Source: CAD feature listing. Evaluate the final solid. Frame: model axes, mm. A direction names the side the tool comes from. Round coordinates to 2 decimals unless told otherwise and drop trailing zeros. Loops run counter-clockwise (first coordinate to the right, second up) from the corner with the lowest first, then second, coordinate; pieces in that order, holes last.
(1) Section C-C, the plane y = 86. Return the cut outline in (x, z).
(2) Section A-A, the plane x = 155. Return the cut outline in (y, z).
(3) Set-up query: faces 1 (the flat face through (202.597, 33, -36)), 2 (the flat face through (32, 73.19, -52)). Return all of +Z, -Z, +X, -X, +Y, -Y with unobstructed straight access to the full face (end or side cutting, diameter ignored); none if empty.
(4) Section B-B, the plane z = 43. Return the cut outline in (x, y).
(5) Mould query, pull axis X, two halves, no side actions, for faces 3 (the cylindrical face through (43.02, 85.71, 2.95)), 4 (the flat face through (62, -31.08, -36)), 5 (the flat face through (-73.991, 33, -36)). Classes: pulls with the +X half, pulls with the -X half, needs draft (parallel to the pull), parting line crosses it, or undercut.
```python
from build123d import *

# Parameters (mm, degrees)
F0_W     = 144.507817924
F0_H     = 104.2701918632
F1_DEPTH = 104.394
F2_DEPTH = 276.86
F3_DEPTH = 132.08
F4_W     = 276.587817924
F4_H     = 276.86
F4_R     = 25.1884721884
F4_R_2   = 24.4502004905
F4_R_3   = 28.2958784433
F4_R_4   = 27.5167719558
F5_DEPTH = 25.4


with BuildPart() as f1:
    # F0 (on Top) → F1 (new body)
    with BuildSketch(Plane.XY):
        with Locations((-1.7366670072, 21.054728888)):
            Rectangle(F0_W, F0_H)
    extrude(amount=F1_DEPTH)

    # F2 (add): a face of the model
    f2_faces = [f1.faces().sort_by_distance(p)[0] for p in [
        (-1.7366670072, 21.054728888, 104.394),
    ]]
    extrude(f2_faces, amount=-F2_DEPTH)

    # F3 (add): a face of the model
    f3_faces = [f1.faces().sort_by_distance(p)[0] for p in [
        (70.5172419548, 21.054728888, -34.036),
    ]]
    extrude(f3_faces, amount=F3_DEPTH)

    # F4 (on face) → F5 (join)
    with BuildSketch(Plane(origin=(0, 73.1898248196, 0), x_dir=(-1, 0, 0), z_dir=(0, 1, 0))):
        with Locations((-64.3033329928, -34.036)):
            Rectangle(F4_W, F4_H)
        with Locations((-170.0846999884, -71.3028535247)):
            Circle(F4_R, mode=Mode.SUBTRACT)
        with Locations((-32.8044444323, -52.5894537568)):
            Circle(F4_R_2, mode=Mode.SUBTRACT)
        with Locations((-163.5096520185, 28.9383083582)):
            Circle(F4_R_3, mode=Mode.SUBTRACT)
        with Locations((-21.1840029806, 19.6925438941)):
            Circle(F4_R_4, mode=Mode.SUBTRACT)
    extrude(amount=F5_DEPTH)


solid = f1.part
```
Output values:
1. outline: (-73.99, -172.47) - (202.6, -172.47) - (202.6, 104.39) - (-73.99, 104.39) - close; hole circle Ø55.03 at (21.18, 19.69); hole circle Ø48.9 at (32.8, -52.59); hole circle Ø56.59 at (163.51, 28.94); hole circle Ø50.38 at (170.08, -71.3)
2. outline: (-31.08, -172.47) - (98.59, -172.47) - (98.59, -91.47) - (73.19, -91.47) - (73.19, -51.13) - (98.59, -51.13) - (98.59, 1.95) - (73.19, 1.95) - (73.19, 55.92) - (98.59, 55.92) - (98.59, 104.39) - (-31.08, 104.39) - close
3. face 1: +Z, -Z, +X, +Y, -Y
3. face 2: +Y
4. outline: (-73.99, -31.08) - (202.6, -31.08) - (202.6, 98.59) - (188.06, 98.59) - (188.06, 73.19) - (138.96, 73.19) - (138.96, 98.59) - (35.81, 98.59) - (35.81, 73.19) - (6.56, 73.19) - (6.56, 98.59) - (-73.99, 98.59) - close
5. face 3: undercut
5. face 4: needs draft
5. face 5: pulls with the -X half
